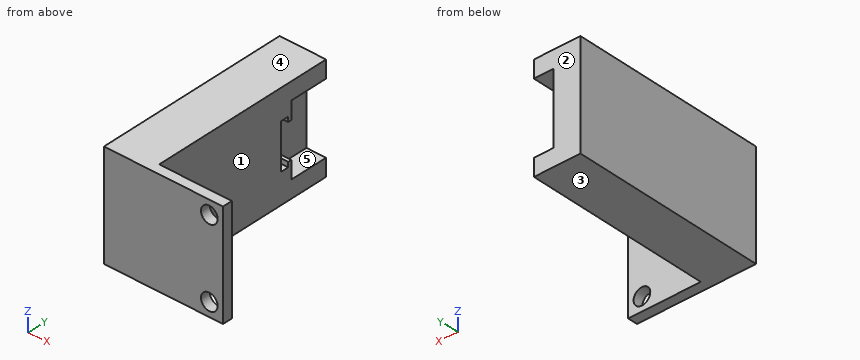
from build123d import *

# Parameters (mm, degrees)
SKETCH1_W            = 84.39
SKETCH1_H            = 54
SKETCH1_R            = 4.25
BOSS_EXTRUDE1_DEPTH  = 100
CUT_EXTRUDE1_DEPTH   = 10
SKETCH3_W            = 36.999403
SKETCH3_H            = 54
CUT_EXTRUDE2_DEPTH   = 95
MIRROR2_COPY_1_DEPTH = 10
CUT_EXTRUDE3_REACH   = 122.054
SKETCH4_W            = 141.405079451
SKETCH4_H            = 141.172887202


with BuildPart() as part:
    # Sketch1 → Boss-Extrude1 (new body)
    with BuildSketch(Plane(origin=(0, 0, 0), x_dir=(1, 0, 0), z_dir=(0, 1, 0))):
        Rectangle(SKETCH1_W, SKETCH1_H)
        with Locations(Location((35.195, 20, 0), (0, 0, 270))):
            Circle(SKETCH1_R, mode=Mode.SUBTRACT)
        with Locations(Location((35.195, -20, 0), (0, 0, 270))):
            Circle(SKETCH1_R, mode=Mode.SUBTRACT)
    extrude(amount=BOSS_EXTRUDE1_DEPTH)

    # Sketch2 → Cut-Extrude1 (cut)
    with BuildSketch(Plane.ZY.offset(42.195)):
        Polygon((-11.65, 78.45), (-9.15, 78.45), (-9.15, 80.267556596), (-18.171447478, 80.267556596), (-18.171447478, 100), (0, 100), (0, 74.25), (-11.65, 74.25), align=None)
    cut_extrude1 = extrude(amount=-CUT_EXTRUDE1_DEPTH, mode=Mode.SUBTRACT)

    # Sketch3 → Cut-Extrude2 (cut)
    with BuildSketch(Plane(origin=(0, 100, 0), x_dir=(1, 0, 0), z_dir=(0, 1, 0))):
        with Locations((23.6952985, 0)):
            Rectangle(SKETCH3_W, SKETCH3_H)
    extrude(amount=-CUT_EXTRUDE2_DEPTH, mode=Mode.SUBTRACT)

    # Mirror1: Cut-Extrude1 across plane
    add(cut_extrude1.mirror(Plane.XY), mode=Mode.SUBTRACT)

    # Mirror2: Cut-Extrude1 across plane
    add(cut_extrude1.mirror(Plane(origin=(-18.4997015, 0, 0), x_dir=(0, 0, 1), z_dir=(1, 0, 0))), mode=Mode.SUBTRACT)

    # Mirror2 copy 1 sketch → Mirror2 copy 1 (cut)
    with BuildSketch(Plane(origin=(5.195597, 0, 0), x_dir=(0, 0, -1), z_dir=(1, 0, 0))):
        Polygon((-11.65, 78.45), (-9.15, 78.45), (-9.15, 80.267556596), (-18.171447478, 80.267556596), (-18.171447478, 100), (0, 100), (0, 74.25), (-11.65, 74.25), align=None)
    extrude(amount=-MIRROR2_COPY_1_DEPTH, mode=Mode.SUBTRACT)

    # Sketch4 → Cut-Extrude3 (cut, up to next)
    with BuildSketch(Plane(origin=(-18.4997015, 0, 0), x_dir=(0, 0, -1), z_dir=(1, 0, 0)), mode=Mode.PRIVATE) as cut_extrude3_sk1:
        with Locations((22.522648123, 44.65957828)):
            Rectangle(SKETCH4_W, SKETCH4_H)
    cut_extrude3_tool1 = extrude(cut_extrude3_sk1.sketch, amount=-CUT_EXTRUDE3_REACH, mode=Mode.PRIVATE) & part.part
    add(cut_extrude3_tool1.solids().sort_by_distance((-18.499701, 44.659578, -22.522648))[0], mode=Mode.SUBTRACT)


solid = part.part
Check sheet for the modelled part. Datum: model origin and axes. Units: mm. Face numbers are marked on the shaded views. A direction names the side the tool comes from. Give positions to 0.01 mm unless a question says otherwise; leave off trailing zeros. Loops run counter-clockwise (first coordinate to the right, second up) from the corner with the lowest first, then second, coordinate; pieces in that order, holes last. Notation, with made-up numbers: M -17,35.5 L 38,35.5 A25 cw 38,63.5 Z; hole C 30,-6 d4. An arc over 180 degrees is marked long. Use a Markdown table: item, result. Add a question column.
Q1. Sectioned sample at B-B, the plane y = 83. Record the cut outline in (x, z).
Q2. Sectioned sample at A-A, the plane z = 20. Record the cut outline in (x, y) (3 decimals), then the cut area to 3 significant figures.
Q3. Sectioned sample at C-C, the plane x = -0.5. Record the cut outline in (y, z), then the cut area to 3 significant figures.
Q4. Scan lines: line 1 along X through (y, z) = (1, 20) (3 decimals); line 2 along X through (y, z) = (44, 14.5); line 3 along Y through (x, z) = (14.5, 5). Record each from-to range of solid material in increasing order. Write a range as [from, to].
Q5. Tool access check on the marked faces 1 and 2. Record the directions out of +Z, -Z, +X, -X, +Y, -Y that give a thin tool (end or side, any length) a straight path to the whole face; none if there is none.
Q6. Mould release check, pull along Z, two halves, no side actions. Record for the marked faces 3, 4 and 5: pulls with the +Z half, pulls with the -Z half, needs draft (parallel to the pull), parting line crosses it, or undercut.
Q7. Sectioned sample at D-D, the plane z = -8. Record the cut outline in (x, y) (3 decimals).
Q8. Go/stop test with flat-tipped pins: pin 1 (2.5 mm diameter, centred on x = -0.5, z = 14.5, fed in from +Y); pin 2 (7.5 mm diameter, centred on y = 86, z = 5, fed in from +X); pin 3 (5 mm diameter, centred on x = 2.5, z = 4.5, fed in from +Y). Record where each tip stops, or that it passes through.
Verdict:
| question | item | result |
|---|---|---|
| 1 | outline | M -18.5,-27 L 5.2,-27 L 5.2,-18.17 L -4.8,-18.17 L -4.8,18.17 L 5.2,18.17 L 5.2,27 L -18.5,27 Z |
| 2 | outline | M -18.5,0 L 30.945,0 L 30.945,5 L 5.196,5 L 5.196,100 L -18.5,100 Z; M 39.445,0 L 42.195,0 L 42.195,5 L 39.445,5 Z |
| 2 | area | 2,510 mm^2 |
| 3 | outline | M 0,-27 L 100,-27 L 100,-18.17 L 80.27,-18.17 L 80.27,-9.15 L 78.45,-9.15 L 78.45,-11.65 L 74.25,-11.65 L 74.25,11.65 L 78.45,11.65 L 78.45,9.15 L 80.27,9.15 L 80.27,18.17 L 100,18.17 L 100,27 L 0,27 Z |
| 3 | area | 4,550 mm^2 |
| 4 | line 1 | [-18.5, 30.945], [39.445, 42.195] |
| 4 | line 2 | [-18.5, 5.2] |
| 4 | line 3 | [0, 5] |
| 5 | face 1 | +Z, -Z, +X, +Y |
| 5 | face 2 | +Z, -Z, +X, -X, +Y |
| 6 | face 3 | pulls with the -Z half |
| 6 | face 4 | pulls with the +Z half |
| 6 | face 5 | undercut |
| 7 | outline | M -18.5,0 L 42.195,0 L 42.195,5 L 5.196,5 L 5.196,74.25 L -4.804,74.25 L -4.804,100 L -18.5,100 Z |
| 8 | pin 1 | y = 80.27 |
| 8 | pin 2 | x = -4.8 |
| 8 | pin 3 | y = 74.25 |
